Autodesk Inventor part; units mm, degrees
ref_plane "YZ Plane" through (0, 0, 0) normal (1, 0, 0) x (0, 1, 0)
ref_plane "XZ Plane" through (0, 0, 0) normal (0, 1, 0) x (-1, 0, 0)
ref_plane "XY Plane" through (0, 0, 0) normal (0, 0, 1) x (1, 0, 0)
sketch "Boceto1" plane through (0, 0, 0) normal (0, 1, 0) x (-1, 0, 0)
  circle A0 centre (0, 0) radius 75
  circle A1 centre (62.5, 0) radius 5
  circle A2 centre (62.5, 0) radius 8
  circle A3 centre (0, 0) radius 13
  circle A4 centre (-31.25, -54.1266) radius 5
  circle A5 centre (-31.25, -54.1266) radius 8
  circle A6 centre (-31.25, 54.1266) radius 5
  circle A7 centre (-31.25, 54.1266) radius 8
  dimension "d0" = 150
  dimension "d1" = 10
  dimension "d2" = 16
  dimension "d3" = 26
  dimension "d4" = 10
  dimension "d5" = 16
  dimension "d6" = 10
  dimension "d7" = 16
extrude "Extrusión1" add sketch "Boceto1" along normal blind 14 contours A0 | A2 | A5 | A7
sketch "Boceto2" plane through (0, 14, 0) normal (0, 1, 0) x (1, 0, 0)
  point P0 (0, 0)
sketch "Boceto3" plane through (0, 14, 0) normal (0, 1, 0) x (1, 0, 0)
  circle A0 centre (0, 0) radius 50.5
  circle A1 centre (-62.5, 0) radius 8
  circle A2 centre (31.25, 54.1266) radius 5
  circle A3 centre (31.25, 54.1266) radius 8
  circle A4 centre (31.25, -54.1266) radius 5
  circle A5 centre (31.25, -54.1266) radius 8
  dimension "d10" = 101
  dimension "d11" = 16
  dimension "d12" = 16
  dimension "d13" = 16
extrude "Extrusión2" cut sketch "Boceto3" against normal blind 10 contours A1 | A2 | A3 | A4 | A5
extrude "Extrusión3" cut sketch "Boceto3" against normal blind 5 contours A0
properties part number "1.1.5.UpperSta.Plate"
The listing builds one solid part. Answer for the finished solid, in the listing's coordinates (mm). A direction names the side the tool comes from. Round coordinates to 2 decimals unless told otherwise and drop trailing zeros. Order: outer loops, then holes, each group sorted by start corner. A loop starts at its lowest first (then second) coordinate and runs counter-clockwise, first axis right, second up. Notation, with made-up numbers: (28.25, 24.5) -> (82.25, 24.5) arc R26 ccw to (82.25, 40.5) -> close; hole circle Ø4 at (50.25, -28). An arc over 180 degrees is marked (long way). Answer as CSV lines item,"result". Start each with the question number.
(1) The part is cut by section C-C (x = 31.25). Determine the outline of the cut face in (y, z), then the cut area to 3 significant figures.
(2) Find the intervals of material crossed by probe 1 along Z at (x, y) = (0, 2.75); probe 2 along Z at (x, y) = (31.25, 7.75); probe 3 along Z at (x, y) = (0, 11.1), in increasing order. Write a range as from..to.
(3) The part is cut by section B-B (x = 0). Determine the outline of the cut face in (y, z), then the cut area to 3 significant figures.
(4) The part is cut by section A-A (z = 0). Determine the outline of the cut face in (x, y).
(5) A tool of negligible diameter and unlimited length cuts with its end or side. For faces 4 (the face through (-57.505, 1.972, -0.22)), 5 (the face through (-10.95, 11.54, 49.3)), from which of +Z, -Z, +X, -X, +Y, -Y can it reach the whole face along a straight path? Write none if from no direction.
(6) The part is cut by section D-D (y = 11). Determine the outline of the cut face in (x, z).
(7) For a pull along Y with two mould halves and no side action, classify faces 1 (the face through (-59, 4, -4)), 2 (the face through (1, 0, -16)), 3 (the face through (32.334, 1.972, -49.245)) as +Y half, -Y half, draft (parallel to the pull), parting line (faces both ways), or undercut.
(8) Flat-ended cylindrical pins translate along their axes: pin 1 Ø4 at (y, z) = (10.5, -39) entering from +X; pin 2 Ø1 at (y, z) = (5.5, -54) entering from -X; pin 3 Ø9 at (x, z) = (31.25, 54.13) entering from +Y; pin 4 Ø13 at (x, z) = (29, -53.5) entering from +Y. Find the tip coordinate at first contact, or state that the pin passes through.
Evaluation:
1,outline,"(0, -68.18) -> (14, -68.18) -> (14, -62.13) -> (4, -62.13) -> (4, -59.13) -> (0, -59.13) -> close; (0, -49.13) -> (4, -49.13) -> (4, -46.13) -> (14, -46.13) -> (14, -39.67) -> (9, -39.67) -> (9, 39.67) -> (14, 39.67) -> (14, 46.13) -> (4, 46.13) -> (4, 49.13) -> (0, 49.13) -> close; (0, 59.13) -> (4, 59.13) -> (4, 62.13) -> (14, 62.13) -> (14, 68.18) -> (0, 68.18) -> close"
1,area,"1,110 mm²"
2,probe 1,"-75..-13, 13..75"
2,probe 2,"-68.18..-62.13, -46.13..46.13, 62.13..68.18"
2,probe 3,"-75..-50.5, 50.5..75"
3,outline,"(0, -75) -> (14, -75) -> (14, -50.5) -> (9, -50.5) -> (9, -13) -> (0, -13) -> close; (0, 13) -> (9, 13) -> (9, 50.5) -> (14, 50.5) -> (14, 75) -> (0, 75) -> close"
3,area,"1,360 mm²"
4,outline,"(-75, 0) -> (-67.5, 0) -> (-67.5, 4) -> (-70.5, 4) -> (-70.5, 14) -> (-75, 14) -> close; (-57.5, 0) -> (-13, 0) -> (-13, 9) -> (-50.5, 9) -> (-50.5, 14) -> (-54.5, 14) -> (-54.5, 4) -> (-57.5, 4) -> close; (13, 0) -> (75, 0) -> (75, 14) -> (50.5, 14) -> (50.5, 9) -> (13, 9) -> close"
5,face 4,"+Y, -Y"
5,face 5,"+Y"
6,outline,"circle Ø150 at (0, 0); hole circle Ø16 at (-62.5, 0); hole circle Ø101 at (0, 0); hole circle Ø16 at (31.25, -54.13); hole circle Ø16 at (31.25, 54.13)"
7,face 1,"+Y half"
7,face 2,"-Y half"
7,face 3,"draft"
8,pin 1,"x = 65.24"
8,pin 2,"x = -52.56"
8,pin 3,"through"
8,pin 4,"y = 14"
